For this review, take the finished solid that the model builds, in its own axes (mm). A direction names the side the tool comes from. Coordinates: 2 decimals unless noted, no trailing zeros. Write each loop counter-clockwise with the first axis right and the second up, starting at its lowest first coordinate (ties: lowest second). Pieces come first, ordered by that corner, then holes. Notation, with made-up numbers: M -38,39 L 8,39 A13 cw 8,62 Z; hole C 53,-40 d4. An arc over 180 degrees is marked long. One line per question, with ' | ' between items.
from build123d import *

# Parameters (mm, degrees)
EXTRUDE_1_DEPTH     = 13
SKETCH_2_R          = 1
SKETCH_2_R_2        = 1.5
CUT_EXTRUDE_1_DEPTH = 22.685248442


with BuildPart() as part:
    # 草图1 → 凸台-拉伸1 (new body)
    with BuildSketch(Plane.XY):
        Polygon((-7.5, 6.5), (-7.5, -4), (7.5, -4), (7.5, 6.5), (11.5, 6.5), (11.5, -6.5), (-11.5, -6.5), (-11.5, 6.5), align=None)
    extrude(amount=EXTRUDE_1_DEPTH)

    # 草图2 → 切除-拉伸1 (cut, through all)
    with BuildSketch(Plane(origin=(0, 6.5, 0), x_dir=(1, 0, 0), z_dir=(0, 1, 0))):
        with Locations(Location((-9.504895382, -2.5, 0), (0, 0, 270))):
            Circle(SKETCH_2_R)
        with Locations(Location((-9.504895382, -10.5, 0), (0, 0, 270))):
            Circle(SKETCH_2_R)
        with Locations(Location((9.5, -2.5, 0), (0, 0, 270))):
            Circle(SKETCH_2_R)
        with Locations(Location((9.5, -10.5, 0), (0, 0, 270))):
            Circle(SKETCH_2_R)
        with Locations(Location((0, -6.5, 0), (0, 0, 270))):
            Circle(SKETCH_2_R_2)
    extrude(amount=-CUT_EXTRUDE_1_DEPTH, mode=Mode.SUBTRACT)


solid = part.part
1. Clearance check with flat-ended pins moving along their axes: P1, Ø1.6, axis at x = 9.5, z = 2.5, coming from the +Y side; P2, Ø3, axis at x = -9.5, z = 2.5, coming from the +Y side; P3, Ø6, axis at x = 1, z = 6.5, coming from the +Y side. State where each tip first meets the part, or that it passes through.
Computed values:
P1: passes through | P2: stops at y = 6.5 | P3: stops at y = -4
2. Take a section at B-B on x = 0. State the section outline as (y, z) points, plus the area to 3 significant figures.
Computed values:
outline: M -6.5,0 L -4,0 L -4,5 L -6.5,5 Z; M -6.5,8 L -4,8 L -4,13 L -6.5,13 Z | area: 25.0 mm2
3. For line 1 along X through (y, z) = (-2.5, 2.5); line 2 along X through (y, z) = (-3.5, 8); line 3 along Z through (x, y) = (10.25, 5.5), list the stretches that pass through material, from the lowest coordinate up.
Computed values:
line 1: x = -11.5 to -10.5, -8.5 to -7.5, 7.5 to 8.5, 10.5 to 11.5 | line 2: x = -11.5 to -7.5, 7.5 to 11.5 | line 3: z = 0 to 1.84, 3.16 to 9.84, 11.16 to 13
4. Draft analysis for pull direction X (two halves, no side actions). For faces 3 (the flat face through (11.5, 0, 6)), 4 (the cylindrical face through (10.49, 0.09, 10.37)), 5 (the flat face through (-10, 6.5, 6)), state which applies: pulls with the +X half, pulls with the -X half, needs draft (parallel to the pull), parting line crosses it, or undercut.
Computed values:
face 3: pulls with the +X half | face 4: undercut | face 5: needs draft
5. Take a section at D-D on z = 6.5. State the section outline as (x, y) points.
Computed values:
outline: M -11.5,-6.5 L -1.5,-6.5 L -1.5,-4 L -7.5,-4 L -7.5,6.5 L -11.5,6.5 Z; M 1.5,-6.5 L 11.5,-6.5 L 11.5,6.5 L 7.5,6.5 L 7.5,-4 L 1.5,-4 Z
6. Machinability: for faces 1 (the flat face through (-2, -4, 6)), 2 (the flat face through (9, 6.5, 6)), which of the approach directions +Z, -Z, +X, -X, +Y, -Y give a long, thin tool a straight path to every point of the face, cutting with its end or side? Answer none if there is none.
Computed values:
face 1: +Z, -Z, +Y | face 2: +Z, -Z, +X, -X, +Y
7. Take a section at C-C on y = 4. State the section outline as (x, z) points.
Computed values:
outline: M -11.5,0 L -7.5,0 L -7.5,13 L -11.5,13 Z; M 7.5,0 L 11.5,0 L 11.5,13 L 7.5,13 Z; hole C -9.5,2.5 d2; hole C -9.5,10.5 d2; hole C 9.5,2.5 d2; hole C 9.5,10.5 d2
8. Take a section at A-A on z = 2.5. State the section outline as (x, y) points.
Computed values:
outline: M -11.5,-6.5 L -10.5,-6.5 L -10.5,6.5 L -11.5,6.5 Z; M -8.5,-6.5 L 8.5,-6.5 L 8.5,6.5 L 7.5,6.5 L 7.5,-4 L -7.5,-4 L -7.5,6.5 L -8.5,6.5 Z; M 10.5,-6.5 L 11.5,-6.5 L 11.5,6.5 L 10.5,6.5 Z
